The model under review builds one solid part; all positions refer to its coordinate system, in mm. A direction names the side the tool comes from. Coordinates: 2 decimals unless noted, no trailing zeros. Order: outer loops, then holes, each group sorted by start corner. A loop starts at its lowest first (then second) coordinate and runs counter-clockwise, first axis right, second up.
```python
from build123d import *

# Parameters (mm, degrees)
CROQUIS1_W              = 135
CROQUIS1_H              = 50
CROQUIS1_R              = 0.85
SALIENTE_EXTRUIR1_DEPTH = 15
CROQUIS2_W              = 135
CROQUIS2_H              = 50
CROQUIS2_R              = 0.85
CROQUIS2_R_2            = 5
SALIENTE_EXTRUIR2_DEPTH = 4
CROQUIS3_R              = 1.75
CORTAR_EXTRUIR1_DEPTH   = 12


with BuildPart() as part:
    # Croquis1 → Saliente-Extruir1 (new body)
    with BuildSketch(Plane.XY):
        with Locations((-0.262377426, 0.111379231)):
            Rectangle(CROQUIS1_W, CROQUIS1_H)
        with Locations((-65.012377426, 22.361379231)):
            Circle(CROQUIS1_R, mode=Mode.SUBTRACT)
        with Locations((-65.012377426, -22.138620769)):
            Circle(CROQUIS1_R, mode=Mode.SUBTRACT)
        with Locations((64.487622574, -22.138620769)):
            Circle(CROQUIS1_R, mode=Mode.SUBTRACT)
        with Locations((64.487622574, 22.361379231)):
            Circle(CROQUIS1_R, mode=Mode.SUBTRACT)
        Polygon((-64.762377426, 17.111379231), (-64.762377426, -16.888620769), (-59.762377426, -21.888620769), (15.089266591, -21.888620769), (15.089266591, 22.111379231), (-59.762377426, 22.111379231), align=None, mode=Mode.SUBTRACT)
        Polygon((64.237622574, 17.111379231), (59.237622574, 22.111379231), (18.089266591, 22.111379231), (18.089266591, -21.888620769), (59.237622574, -21.888620769), (64.237622574, -16.888620769), align=None, mode=Mode.SUBTRACT)
    extrude(amount=SALIENTE_EXTRUIR1_DEPTH)

    # Croquis2 → Saliente-Extruir2 (add)
    with BuildSketch(Plane.XY.offset(15)):
        with Locations((-0.262377426, 0.111379231)):
            Rectangle(CROQUIS2_W, CROQUIS2_H)
        with Locations((-65.012377426, 22.361379231)):
            Circle(CROQUIS2_R, mode=Mode.SUBTRACT)
        with Locations((64.487622574, 22.361379231)):
            Circle(CROQUIS2_R, mode=Mode.SUBTRACT)
        with Locations((64.487622574, -22.138620769)):
            Circle(CROQUIS2_R, mode=Mode.SUBTRACT)
        with Locations((-65.012377426, -22.138620769)):
            Circle(CROQUIS2_R, mode=Mode.SUBTRACT)
        with Locations((-29.126949829, -9.66737546)):
            Circle(CROQUIS2_R_2, mode=Mode.SUBTRACT)
        Polygon((18.089266591, 22.111379231), (18.089266591, -21.888620769), (59.237622574, -21.888620769), (64.237622574, -16.888620769), (64.237622574, 17.111379231), (59.237622574, 22.111379231), align=None, mode=Mode.SUBTRACT)
    extrude(amount=SALIENTE_EXTRUIR2_DEPTH)

    # Croquis3 → Cortar-Extruir1 (cut)
    with BuildSketch(Plane.XY.offset(19)):
        with Locations((64.487622574, 22.361379231)):
            Circle(CROQUIS3_R)
        with Locations((64.487622574, -22.138620769)):
            Circle(CROQUIS3_R)
        with Locations((-65.012377426, -22.138620769)):
            Circle(CROQUIS3_R)
        with Locations((-65.012377426, 22.361379231)):
            Circle(CROQUIS3_R)
    extrude(amount=-CORTAR_EXTRUIR1_DEPTH, mode=Mode.SUBTRACT)


solid = part.part
```
(1) We need section B-B, the plane x = 24. Write out the cut boundary in (y, z).
A:
outline: (-24.89, 0) - (-21.89, 0) - (-21.89, 19) - (-24.89, 19) - close; (22.11, 0) - (25.11, 0) - (25.11, 19) - (22.11, 19) - close
(2) Draft analysis for pull direction Y (two halves, no side actions). For faces 1 (the face through (-1, 25.111, 9)), 2 (the face through (-63.343, -21.613, 13.084)), 3 (the face through (-16, 0, 19)), state which applies: released by +Y, released by -Y, zero draft, split by the parting line, or undercut.
A:
face 1: released by +Y
face 2: undercut
face 3: zero draft
(3) We need section D-D, the plane z = 2.5. Write out the cut boundary in (x, y).
A:
outline: (-67.76, -24.89) - (67.24, -24.89) - (67.24, 25.11) - (-67.76, 25.11) - close; hole circle Ø1.7 at (-65.01, -22.14); hole circle Ø1.7 at (-65.01, 22.36); hole (-64.76, -16.89) - (-59.76, -21.89) - (15.09, -21.89) - (15.09, 22.11) - (-59.76, 22.11) - (-64.76, 17.11) - close; hole (18.09, -21.89) - (59.24, -21.89) - (64.24, -16.89) - (64.24, 17.11) - (59.24, 22.11) - (18.09, 22.11) - close; hole circle Ø1.7 at (64.49, -22.14); hole circle Ø1.7 at (64.49, 22.36)
(4) Machinability: for faces 4 (the face through (67.238, 0, 9)), 5 (the face through (15.089, 0, 7)), 6 (the face through (39, 22.111, 9)), 7 (the face through (66.157, 22.887, 13.084)), which of the approach directions +Z, -Z, +X, -X, +Y, -Y give a long, thin tool a straight path to every point of the face, cutting with its end or side? Answer none if there is none.
A:
face 4: +Z, -Z, +X, +Y, -Y
face 5: -Z
face 6: +Z, -Z
face 7: +Z
(5) Wall thickness on probe 1 along X at (y, z) = (-11.5, 10); probe 2 along Y at (x, z) = (12.5, 7); probe 3 along X at (y, z) = (0, 18.25): over which ranges is each line inside the solid? List them lowest first.
A:
probe 1: x = -67.76 to -64.76, 15.09 to 18.09, 64.24 to 67.24
probe 2: y = -24.89 to -21.89, 22.11 to 25.11
probe 3: x = -67.76 to 18.09, 64.24 to 67.24
(6) For pin 1 Ø22 at (x, y) = (-21.5, 2.5) entering from -Z; pin 2 Ø1.8 at (x, y) = (-64.5, 22.5) entering from +Z, all flat-tipped, find the tip position at first contact; note any pin that passes through.
A:
pin 1: stops at z = 15
pin 2: stops at z = 7
(7) We need section A-A, the plane y = 14. Write out the cut boundary in (x, z), and give its area (3 significant figures).
A:
outline: (-67.76, 0) - (-64.76, 0) - (-64.76, 15) - (15.09, 15) - (15.09, 0) - (18.09, 0) - (18.09, 19) - (-67.76, 19) - close; (64.24, 0) - (67.24, 0) - (67.24, 19) - (64.24, 19) - close
area: 490 mm2
(8) We need section C-C, the plane y = -13.5. Write out the cut boundary in (x, z), and give its area (3 significant figures).
A:
outline: (-67.76, 0) - (-64.76, 0) - (-64.76, 15) - (-32.34, 15) - (-32.34, 19) - (-67.76, 19) - close; (-25.92, 15) - (15.09, 15) - (15.09, 0) - (18.09, 0) - (18.09, 19) - (-25.92, 19) - close; (64.24, 0) - (67.24, 0) - (67.24, 19) - (64.24, 19) - close
area: 465 mm2
